Here's how the part is built. I have some questions about the finished solid (model axes, mm). Face numbers are marked on the shaded views. Round coordinates to 2 decimals unless told otherwise and drop trailing zeros. Loops run counter-clockwise (first coordinate to the right, second up) from the corner with the lowest first, then second, coordinate; pieces in that order, holes last. Notation, with made-up numbers: M 25.25,68.25 L 73.25,68.25 A11 cw 73.25,80.25 Z; hole C 62.25,-1.5 d4. An arc over 180 degrees is marked long. Write item = value, one per line. Start each with the question number.
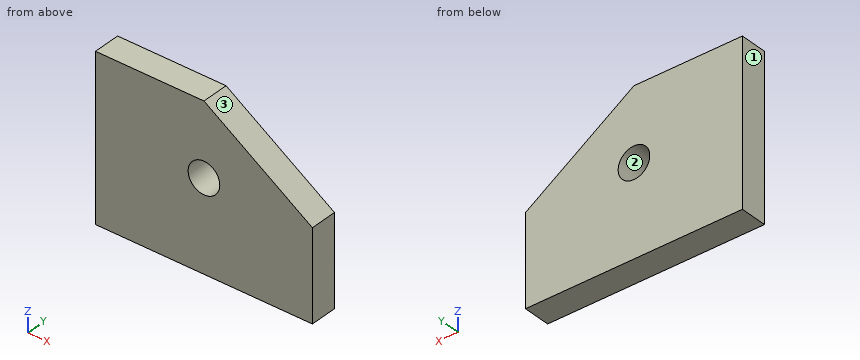
from build123d import *

# Parameters (mm, degrees)
PAD_DEPTH    = 19.05
SKETCH001_R  = 11.1125
POCKET_DEPTH = 19.051


with BuildPart() as part:
    # Sketch → Pad (new body)
    with BuildSketch(Plane.XZ):
        Polygon((-76.2, -63.5), (-76.2, 50.8), (0, 50.8), (76.2, 0), (76.2, -63.5), align=None)
    extrude(amount=PAD_DEPTH)

    # Sketch001 (on Face6 of Pad) → Pocket (cut, through all)
    with BuildSketch(Plane(origin=(0, 0, 0), x_dir=(1, 0, 0), z_dir=(0, 1, 0))):
        Circle(SKETCH001_R)
    extrude(amount=-POCKET_DEPTH, mode=Mode.SUBTRACT)


solid = part.part
Item 1: We'd pull the mould along Z, two halves only. Please class the marked faces 1, 2 and 3: released by +Z, released by -Z, zero draft, split by the parting line, or undercut.
Item 2: I want a section at B-B, the plane x = -3.5. List the corners of the cut face in (y, z) for me, then the cut area to 3 significant figures.
Item 3: I want a section at D-D, the plane z = 42.5. List the corners of the cut face in (x, y) for me.
Item 4: Will this pin go through, and if not, where does the flat tip stop? pin 1 Ø6 at (x, y) = (40, -2.5) entering from +Z.
Item 5: I want a section at A-A, the plane z = 4.5. List the corners of the cut face in (x, y) for me.
Item 6: Please list where these lines run through material, in increasing order: line 1 (X direction, y = -3.75, z = 0); line 2 (Z direction, x = 0, y = -9); line 3 (Z direction, x = -4, y = -1.5). Write a range as [from, to].
Item 7: I want a section at C-C, the plane y = -11.5. List the corners of the cut face in (x, z) for me (1 decimal).
Worked out:
q1.face_1 = zero draft
q1.face_2 = undercut
q1.face_3 = released by +Z
q2.outline = M -19.05,-63.5 L 0,-63.5 L 0,-10.55 L -19.05,-10.55 Z; M -19.05,10.55 L 0,10.55 L 0,50.8 L -19.05,50.8 Z
q2.area = 1,780 mm2
q3.outline = M -76.2,-19.05 L 12.45,-19.05 L 12.45,0 L -76.2,0 Z
q4.pin_1 = 26.13
q5.outline = M -76.2,-19.05 L -10.16,-19.05 L -10.16,0 L -76.2,0 Z; M 10.16,-19.05 L 69.45,-19.05 L 69.45,0 L 10.16,0 Z
q6.line_1 = [-76.2, -11.11], [11.11, 76.2]
q6.line_2 = [-63.5, -11.11], [11.11, 50.8]
q6.line_3 = [-63.5, -10.37], [10.37, 50.8]
q7.outline = M -76.2,-63.5 L 76.2,-63.5 L 76.2,0 L 0,50.8 L -76.2,50.8 Z; hole C 0,0 d22.2
